Check sheet for the modelled part. Datum: model origin and axes. Units: mm. A direction names the side the tool comes from. Coordinates: 2 decimals unless noted, no trailing zeros. Loops run counter-clockwise (first coordinate to the right, second up) from the corner with the lowest first, then second, coordinate; pieces in that order, holes last. Notation, with made-up numbers: (81, -6) -> (110, -6) arc R34 ccw to (110, 28) -> close; hole circle Ø5 at (59.25, 50.5). An arc over 180 degrees is marked (long way). Use CSV: the item, a comma, the result in double quotes.
```python
from build123d import *

# Parameters (mm, degrees)
SKETCH2_R           = 31.75
BOSS_EXTRUDE1_DEPTH = 158.75
SKETCH3_R           = 28.575
BOSS_EXTRUDE2_DEPTH = 19.05
SKETCH4_R           = 25.4
CUT_EXTRUDE1_DEPTH  = 6.35
SKETCH5_R           = 6.35
CUT_EXTRUDE2_DEPTH  = 5.08
DRAFT2_ANGLE        = 45


# Read off the part's stored shape, not the designer's step: Draft3, Shell1
with BuildPart() as part:
    # Sketch2 → Boss-Extrude1 (new body)
    with BuildSketch(Plane(origin=(0, 0, 0), x_dir=(1, 0, 0), z_dir=(0, 1, 0))):
        with Locations(Location((0, 0, 0), (0, 0, 90))):
            Circle(SKETCH2_R)
    extrude(amount=BOSS_EXTRUDE1_DEPTH)

    # Sketch3 → Boss-Extrude2 (add)
    with BuildSketch(Plane(origin=(0, 158.75, 0), x_dir=(1, 0, 0), z_dir=(0, 1, 0))):
        with Locations(Location((0, 0, 0), (0, 0, 90))):
            Circle(SKETCH3_R)
    extrude(amount=BOSS_EXTRUDE2_DEPTH)

    # Sketch4 → Cut-Extrude1 (cut)
    with BuildSketch(Plane.XZ):
        with Locations(Location((0, 0, 0), (0, 0, 270))):
            Circle(SKETCH4_R)
    extrude(amount=-CUT_EXTRUDE1_DEPTH, mode=Mode.SUBTRACT)

    # Sketch5 → Cut-Extrude2 (cut)
    with BuildSketch(Plane.XZ.offset(-6.35)):
        with Locations(Location((0, 0, 0), (0, 0, 270))):
            Circle(SKETCH5_R)
    extrude(amount=-CUT_EXTRUDE2_DEPTH, mode=Mode.SUBTRACT)

    # Draft2
    draft2_faces = [part.faces().sort_by_distance(p)[0] for p in [
        (0, 3.175, 25.4),
    ]]
    draft(draft2_faces, Plane(origin=(0, 0, 0), x_dir=(0, 0, -1), z_dir=(0, -1, 0)), DRAFT2_ANGLE)

    # Draft3 outline → Draft3 (revolve)
    with BuildSketch(Plane.XY):
        Polygon((6.35, 6.35), (6.35, 11.43), (0, 11.43), (0, 10.016174209), align=None)
    revolve(axis=Axis((0, 0, 0), (0, 1, 0)))

    # Shell1 outline → Shell1 (revolve, cut)
    with BuildSketch(Plane.XY):
        Polygon((29.21, 156.21), (26.035, 156.21), (26.035, 177.8), (0, 177.8), (0, 15.882052944), (7.711181898, 11.43), (21.154204897, 11.43), (27.504204897, 5.08), (29.21, 5.08), align=None)
    revolve(axis=Axis((0, 0, 0), (0, 1, 0)), mode=Mode.SUBTRACT)


solid = part.part
```
1) Cross-section at A-A on y = 115. Record the boundary of the cut face in (x, z), and give its area (3 significant figures).
Answer below:
outline,"circle Ø63.5 at (0, 0); hole circle Ø58.42 at (0, 0)"
area,"486 mm²"
2) Thickness scan on line 1 along Y through (x, z) = (-28.5, 5.5); line 2 along X through (y, z) = (81, 0); line 3 along Y through (x, z) = (2, 26.5). Record the ranges inside material, lowest first. Write a range as from..to.
Answer below:
line 1,"y = 0..5.08, 156.21..158.75"
line 2,"x = -31.75..-29.21, 29.21..31.75"
line 3,"y = 0..6.01, 156.21..177.8"
3) Draft check along X on faces 1 (the flat face through (-4.9, 158.75, 28.4)), 2 (the flat face through (-20, 156.21, 17)), 3 (the cylindrical face through (30.995, 78.264, 6.883)). Enter one of: released by +X, released by -X, zero draft, split by the parting line, or undercut.
Answer below:
face 1,"zero draft"
face 2,"undercut"
face 3,"split by the parting line"
4) Access from +Z, -Z, +X, -X, +Y, -Y to the whole of each face (thin tool, end or side, straight path). Record for faces 4 (the cylindrical face through (-3.389, 167.156, -25.813)), 5 (the conical face through (-5, 11, 21)), 6 (the flat face through (5, 6.35, 5)).
Answer below:
face 4,"+Y"
face 5,"none"
face 6,"-Y"
5) Go/stop test with flat-tipped pins: pin 1 Ø12 at (x, y) = (9, 139) entering from -Z; pin 2 Ø12.5 at (x, z) = (1, 2) entering from +Y; pin 3 Ø11.5 at (x, z) = (-6, -8) entering from -Y. Record where each tip stops, or that it passes through.
Answer below:
pin 1,"stops at z = -31.61"
pin 2,"stops at y = 15.88"
pin 3,"stops at y = 6.35"
